Here's how the part is built. I have some questions about the finished solid (model axes, mm). Face numbers are marked on the shaded views. A direction names the side the tool comes from. Round coordinates to 2 decimals unless told otherwise and drop trailing zeros. Loops run counter-clockwise (first coordinate to the right, second up) from the corner with the lowest first, then second, coordinate; pieces in that order, holes last. Notation, with made-up numbers: (-1, 7.5) - (45, 7.5) arc R26 cw to (45, 25.5) - close; hole circle Ø1 at (73.25, 25.5). An arc over 180 degrees is marked (long way). Answer as a JSON object with one key per item and string values. Group by question number.
1) Which directions (+Z, -Z, +X, -X, +Y, -Y) give clear straight access to the entire face, cutting with the end or side of a thin tool? Please do the marked faces 1 and 2.
2) If I drill on line 1 along X through (y, z) = (-1.75, 13); line 2 along Y through (x, z) = (-24, 8.5); line 3 along Z through (x, y) = (23.5, 4.5), over which ranges is the centre line in solid material (lowest first)? Write a range as [from, to].
3) I want a section at C-C, the plane y = 3.25. Please give me the cut outline in (x, z).
4) I want a section at A-A, the plane x = -24. Please give me the cut outline in (y, z), then the cut area to 3 significant figures.
5) If we mould it in two halves opening along Z, with no side actions, what happens to the marked faces 3, 4, 5 and 6? For each: pulls with the +Z half, pulls with the -Z half, needs draft (parallel to the pull), parting line crosses it, or undercut.
Autodesk Inventor part; units mm, degrees
ref_plane "YZ Plane" through (0, 0, 0) normal (1, 0, 0) x (0, 1, 0)
ref_plane "XZ Plane" through (0, 0, 0) normal (0, 1, 0) x (-1, 0, 0)
ref_plane "XY Plane" through (0, 0, 0) normal (0, 0, 1) x (1, 0, 0)
sketch "Sketch1" plane through (0, 0, 0) normal (0, 0, 1) x (1, 0, 0)
  line L0 (-30, 7.5) -> (30, 7.5)
  line L1 (30, 7.5) -> (30, -7.5)
  line L2 (30, -7.5) -> (-30, -7.5)
  line L3 (-30, -7.5) -> (-30, 7.5)
  circle A0 centre (-24, 0) radius 2.5
  point P0 (0, 0)
  point P1 (0, 7.5)
  point P2 (-30, 0)
  dimension "d0" = 5
  dimension "d1" = 6
  dimension "d2" = 15
  dimension "d3" = 60
extrude "Extrusion1" add sketch "Sketch1" along normal blind 35
sketch "Sketch2" plane through (-30, -7.5, 0) normal (0, -1, 0) x (1, 0, 0)
  circle A0 centre (38.5, 8) radius 17.9938
  arc A1 (38.5, 27.5) -> (56.2834, 0) centre (38.5, 8) ccw
  line L0 (38.5, 27.5) -> (60, 27.5)
  line L1 (60, 0) -> (60, 35)
  line L2 (0, 0) -> (60, 0)
  point P0 (30, 0)
  point P1 (20.7166, 0)
  dimension "d6" = 39
extrude "Extrusion2" cut sketch "Sketch2" against normal through all contours A0 L2 | A0 L2 A1 L0 L1 picked at (33.6467, 10.9183)
fillet "Fillet1" radius 7.5 4 edges at (-30, 7.5, 17.5) (-30, -7.5, 17.5) (30, -7.5, 31.25) (30, 7.5, 31.25)
properties part number "0008-30-009"
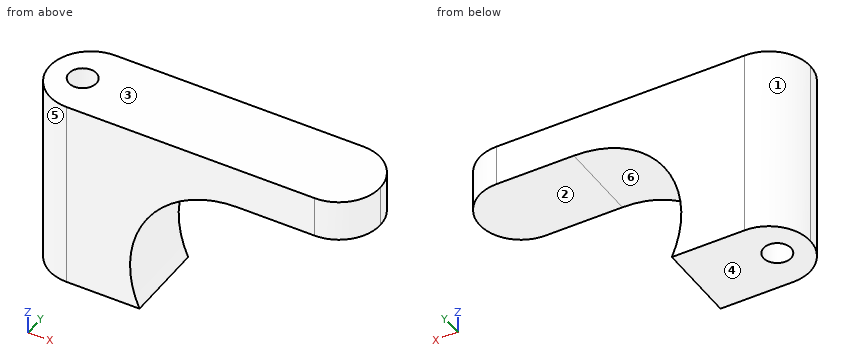
Outcome:
{
 "1": {"face 1": "+Z, -Z, -X, +Y", "face 2": "-Z, +X, +Y, -Y"},
 "2": {"line 1": "[-29.79, -25.79], [-22.21, -10.35]", "line 2": "[-7.35, -2.5], [2.5, 7.35]", "line 3": "[27.5, 35]"},
 "3": {"outline": "(-29.26, 0) - (-9.28, 0) arc R19.5 cw to (8.5, 27.5) - (29.26, 27.5) - (29.26, 35) - (-29.26, 35) - close"},
 "4": {"outline": "(-7.35, 0) - (-2.5, 0) - (-2.5, 35) - (-7.35, 35) - close; (2.5, 0) - (7.35, 0) - (7.35, 35) - (2.5, 35) - close", "area": "339 mm^2"},
 "5": {"face 3": "pulls with the +Z half", "face 4": "pulls with the -Z half", "face 5": "needs draft", "face 6": "undercut"}
}
